Input: part model. Units: mm. Frame: model coordinates. A direction names the side the tool comes from. Give positions to 0.01 mm unless a question says otherwise; leave off trailing zeros. Loops run counter-clockwise (first coordinate to the right, second up) from the corner with the lowest first, then second, coordinate; pieces in that order, holes last. Notation, with made-up numbers: (25, -16) - (29, -16) arc R11 cw to (29, -10) - close; hole circle Ø7 at (-7, 21). An arc over 180 degrees is marked (long way). Answer as a JSON object with one key per item and string values.
from build123d import *

# Parameters (mm, degrees)
F0_W     = 110
F0_H     = 31.75
F1_DEPTH = 6
F2_W     = 110
F2_H     = 6
F3_DEPTH = 25.4
F5_DEPTH = 31.401


with BuildPart() as f1:
    # F0 (on Top) → F1 (new body)
    with BuildSketch(Plane.XY):
        with Locations((55, 15.875)):
            Rectangle(F0_W, F0_H)
    extrude(amount=F1_DEPTH)

    # F2 (on face) → F3 (join)
    with BuildSketch(Plane.XY.offset(6)):
        with Locations((55, 3)):
            Rectangle(F2_W, F2_H)
    extrude(amount=F3_DEPTH)

    # F4 (on face) → F5 (cut, through all)
    with BuildSketch(Plane(origin=(0, 0, 0), x_dir=(1, 0, 0), z_dir=(0, 0, -1))):
        with BuildLine():
            ThreePointArc((54.5588247478, -23.749), (57.3872518725, -22.5774271247), (58.5588247478, -19.749))
            ThreePointArc((58.5588247478, -19.749), (57.3872518725, -16.9205728753), (54.5588247478, -15.749))
            Line((54.5588247478, -15.749), (54.5588247478, -19.749))
            Line((54.5588247478, -19.749), (54.5588247478, -23.749))
        make_face()
        with BuildLine():
            ThreePointArc((54.5588247478, -15.749), (57.3872518725, -16.9205728753), (58.5588247478, -19.749))
            ThreePointArc((58.5588247478, -19.749), (57.3872518725, -22.5774271247), (54.5588247478, -23.749))
            Line((54.5588247478, -23.749), (110, -23.749))
            Line((110, -23.749), (110, -15.749))
            Line((110, -15.749), (54.5588247478, -15.749))
        make_face()
        with BuildLine():
            Line((54.5588247478, -19.749), (54.5588247478, -15.749))
            ThreePointArc((54.5588247478, -15.749), (50.5588247478, -19.749), (54.5588247478, -23.749))
            Line((54.5588247478, -23.749), (54.5588247478, -19.749))
        make_face()
    extrude(amount=-F5_DEPTH, mode=Mode.SUBTRACT)


solid = f1.part
Item 1: Cut plane D-D (x = 14). Return loops of the section in (y, z).
Geometry check:
{"outline": "(0, 0) - (31.75, 0) - (31.75, 6) - (6, 6) - (6, 31.4) - (0, 31.4) - close"}
Item 2: Cut plane C-C (y = 11). Return loops of the section in (x, z), then the cut area to 3 significant figures.
Geometry check:
{"outline": "(0, 0) - (110, 0) - (110, 6) - (0, 6) - close", "area": "660 mm2"}
Item 3: Cut plane B-B (z = 5). Return loops of the section in (x, y).
Geometry check:
{"outline": "(0, 0) - (110, 0) - (110, 15.75) - (54.56, 15.75) arc R4 cw to (54.56, 23.75) - (110, 23.75) - (110, 31.75) - (0, 31.75) - close"}
Item 4: Contact query for flat-ended pins moving along their axis: P1, Ø1, axis at x = 73.5, z = 7, coming from the +Y side; P2, Ø3, axis at x = 22, y = 11, coming from the +Z side. Output: stop coordinate, or through.
Geometry check:
{"P1": "stops at y = 6", "P2": "stops at z = 6"}
Item 5: Access query for faces 1 (the face through (54, 6, 19)), 2 (the face through (54, 13, 0)). Directions: +Z, -Z, +X, -X, +Y, -Y. A direction counts if a zero-diameter tool reaches every point of the face in a straight line with its end or side. Return the directions, or none.
Geometry check:
{"face 1": "+Z, +X, -X, +Y", "face 2": "-Z, +X, -X, +Y, -Y"}
Item 6: Mould query, pull axis Y, two halves, no side actions, for faces 3 (the face through (83, 15.749, 3)), 4 (the face through (82, 23.749, 3)), 5 (the face through (0, 9, 5)), 6 (the face through (54, 31.75, 3)). Classes: released by +Y, released by -Y, zero draft, split by the parting line, or undercut.
Geometry check:
{"face 3": "undercut", "face 4": "undercut", "face 5": "zero draft", "face 6": "released by +Y"}
Item 7: Cut plane A-A (x = 88.5). Return loops of the section in (y, z).
Geometry check:
{"outline": "(0, 0) - (15.75, 0) - (15.75, 6) - (6, 6) - (6, 31.4) - (0, 31.4) - close; (23.75, 0) - (31.75, 0) - (31.75, 6) - (23.75, 6) - close"}
Item 8: Material intervals for line 1 (Y direction, x = 8, z = 13.5); line 2 (Y direction, x = 78, z = 5.5), sorted ascending. Write a range as [from, to].
Geometry check:
{"line 1": "y = [0, 6]", "line 2": "y = [0, 15.75], [23.75, 31.75]"}
